Here's how the part is built. I have some questions about the finished solid (model axes, mm). A direction names the side the tool comes from. Give positions to 0.01 mm unless a question says otherwise; leave off trailing zeros. Loops run counter-clockwise (first coordinate to the right, second up) from the corner with the lowest first, then second, coordinate; pieces in that order, holes last.
Q1. For faces 1 (the face through (6.05, -14, 0)), 2 (the face through (-4, 11.55, -3)), 3 (the face through (6.25, -14, 0)), 4 (the face through (-6.25, -14, 0)), which set-ups out of +Z, -Z, +X, -X, +Y, -Y let a thin tool reach every point of the face, with its end or its side?
Q2. If we section it at D-D (y = 18): Please give me the cut outline in (x, z).
Q3. Will these pins go through, and if not, where does the flat tip stop? P1, Ø5, axis at y = -4, z = -3.5, coming from the +X side; P2, Ø1.6, axis at x = 4.33, z = 2.5, coming from the +Y side; P3, Ø2, axis at y = -14.5, z = 0, coming from the +X side.
Q4. I need wall thicknesses on line 1 (Y direction, x = 5.5, z = 2); line 2 (X direction, y = 12.7, z = 2.5); line 3 (Y direction, x = -3.75, z = -2.5). Which ranges of each line are inside material? Lowest first, please.
Q5. If we section it at C-C (y = 12): Please give me the cut outline in (x, z), plus the area to 3 significant figures.
Q6. If we section it at B-B (z = 0): Please give me the cut outline in (x, y), plus the area to 3 significant figures.
Q7. If we section it at A-A (x = 0): Please give me the cut outline in (y, z), plus the area to 3 significant figures.
Q8. We'd pull the mould along Z, two halves only. Please class faces 5 (the face through (0.225, 19.583, 0.715)), 6 (the face through (-6.05, -14, 0)), 7 (the face through (4, 11.55, 2)), 8 (the face through (0, 0, 6)): +Z half, -Z half, draft (parallel to the pull), parting line (faces both ways), or undercut.
from build123d import *

# Parameters (mm, degrees)
BOSS_EXTRUDE1_DEPTH = 13.45
SKETCH2_R           = 2.35
BOSS_EXTRUDE2_DEPTH = 1.4
SKETCH3_R           = 0.75
BOSS_EXTRUDE5_DEPTH = 9.6
SKETCH4_W           = 0.2
SKETCH4_H           = 4.7
BOSS_EXTRUDE6_DEPTH = 1.9
SKETCH5_R           = 1
CUT_EXTRUDE1_DEPTH  = 1.9


with BuildPart() as part:
    # Sketch1 → Boss-Extrude1 (new, symmetric)
    with BuildSketch(Plane(origin=(0, 0, 0), x_dir=(1, 0, 0), z_dir=(0, 1, 0))):
        with BuildLine():
            Line((-4.905354218, 6), (4.905354218, 6))
            ThreePointArc((4.905354218, 6), (7.75, 0), (4.905354218, -6))
            Line((4.905354218, -6), (-4.905354218, -6))
            ThreePointArc((-4.905354218, -6), (-7.75, 0), (-4.905354218, 6))
        make_face()
    extrude(amount=BOSS_EXTRUDE1_DEPTH, both=True)

    # Sketch2 → Boss-Extrude2 (add)
    with BuildSketch(Plane(origin=(0, 13.45, 0), x_dir=(1, 0, 0), z_dir=(0, 1, 0))):
        with Locations(Location((0, 0, 0), (0, 0, 270))):
            Circle(SKETCH2_R)
    extrude(amount=BOSS_EXTRUDE2_DEPTH)

    # Sketch3 → Boss-Extrude5 (add)
    with BuildSketch(Plane(origin=(0, 14.85, 0), x_dir=(1, 0, 0), z_dir=(0, 1, 0))):
        with Locations(Location((0, 0, 0), (0, 0, 270))):
            Circle(SKETCH3_R)
    extrude(amount=BOSS_EXTRUDE5_DEPTH)

    # Sketch4 → Boss-Extrude6 (add)
    with BuildSketch(Plane.XZ.offset(13.45)):
        with Locations((-6.15, 0)):
            Rectangle(SKETCH4_W, SKETCH4_H)
        with Locations((6.15, 0)):
            Rectangle(SKETCH4_W, SKETCH4_H)
    extrude(amount=BOSS_EXTRUDE6_DEPTH)

    # Sketch5 → Cut-Extrude1 (cut)
    with BuildSketch(Plane(origin=(0, 13.45, 0), x_dir=(1, 0, 0), z_dir=(0, 1, 0))):
        with Locations(Location((-4.330127019, 2.5, 0), (0, 0, 270))):
            Circle(SKETCH5_R)
        with Locations(Location((4.330127019, -2.5, 0), (0, 0, 270))):
            Circle(SKETCH5_R)
    extrude(amount=-CUT_EXTRUDE1_DEPTH, mode=Mode.SUBTRACT)


solid = part.part
Check sheet entries:
1. face 1: +Z, -Z, -Y
1. face 2: +Y
1. face 3: +Z, -Z, +X, -Y
1. face 4: +Z, -Z, -X, -Y
2. outline: circle Ø1.5 at (0, 0)
3. P1: stops at x = 7.69
3. P2: stops at y = 11.55
3. P3: stops at x = 6.25
4. line 1: y = -13.45 to 13.45
4. line 2: x = -7.34 to 3.33, 5.33 to 7.34
4. line 3: y = -13.45 to 11.55
5. outline: (-4.91, -6) - (4.91, -6) arc R7.75 ccw to (4.91, 6) - (-4.91, 6) arc R7.75 ccw to start; hole circle Ø2 at (-4.33, -2.5); hole circle Ø2 at (4.33, 2.5)
5. area: 159 mm2
6. outline: (-7.75, -13.45) - (-6.25, -13.45) - (-6.25, -15.35) - (-6.05, -15.35) - (-6.05, -13.45) - (6.05, -13.45) - (6.05, -15.35) - (6.25, -15.35) - (6.25, -13.45) - (7.75, -13.45) - (7.75, 13.45) - (2.35, 13.45) - (2.35, 14.85) - (0.75, 14.85) - (0.75, 24.45) - (-0.75, 24.45) - (-0.75, 14.85) - (-2.35, 14.85) - (-2.35, 13.45) - (-7.75, 13.45) - close
6. area: 439 mm2
7. outline: (-13.45, -6) - (13.45, -6) - (13.45, -2.35) - (14.85, -2.35) - (14.85, -0.75) - (24.45, -0.75) - (24.45, 0.75) - (14.85, 0.75) - (14.85, 2.35) - (13.45, 2.35) - (13.45, 6) - (-13.45, 6) - close
7. area: 344 mm2
8. face 5: parting line
8. face 6: draft
8. face 7: undercut
8. face 8: +Z half
